Here's how the part is built. I have some questions about the finished solid (model axes, mm). A direction names the side the tool comes from. Give positions to 0.01 mm unless a question says otherwise; leave off trailing zeros. Write each loop counter-clockwise with the first axis right and the second up, starting at its lowest first coordinate (ties: lowest second). Pieces come first, ordered by that corner, then holes. Notation, with made-up numbers: M 54.25,57 L 109.25,57 A25 ccw 109.25,84 Z; hole C 87,-17 d9. An arc over 180 degrees is marked long. Use one line per item in the form item = value. Start each with the question number.
from build123d import *

# Parameters (mm, degrees)
CROQUIS1_R              = 5
CROQUIS1_R_2            = 2.2
SALIENTE_EXTRUIR1_DEPTH = 8
CORTAR_EXTRUIR1_DEPTH   = 26
CROQUIS1_3_R            = 5
CROQUIS1_3_R_2          = 2.65
SALIENTE_EXTRUIR2_DEPTH = 13


with BuildPart() as part:
    # Croquis1 → Saliente-Extruir1 (new body)
    with BuildSketch(Plane(origin=(0, 0, 0), x_dir=(1, 0, 0), z_dir=(0, 1, 0))):
        with BuildLine():
            ThreePointArc((-25, 7), (-24.121320344, 9.121320344), (-22, 10))
            Line((-22, 10), (22, 10))
            ThreePointArc((22, 10), (24.121320344, 9.121320344), (25, 7))
            Line((25, 7), (25, -7))
            ThreePointArc((25, -7), (24.121320344, -9.121320344), (22, -10))
            Line((22, -10), (-22, -10))
            ThreePointArc((-22, -10), (-24.121320344, -9.121320344), (-25, -7))
            Line((-25, -7), (-25, 7))
        make_face()
        with Locations((14.5, 0)):
            Circle(CROQUIS1_R, mode=Mode.SUBTRACT)
        with Locations((-7.5, 0)):
            Circle(CROQUIS1_R_2, mode=Mode.SUBTRACT)
        with Locations((-17.5, 0)):
            Circle(CROQUIS1_R_2, mode=Mode.SUBTRACT)
    extrude(amount=SALIENTE_EXTRUIR1_DEPTH)

    # Croquis2 → Cortar-Extruir1 (cut)
    with BuildSketch(Plane.XY.offset(10)):
        Polygon((4, 8), (5.004091629, 6.995908371), (27.295002856, 6.995908371), (27.295002856, 8), align=None)
    extrude(amount=-CORTAR_EXTRUIR1_DEPTH, mode=Mode.SUBTRACT)

    # Croquis1_3 → Saliente-Extruir2 (add)
    with BuildSketch(Plane(origin=(0, 0, 0), x_dir=(1, 0, 0), z_dir=(0, 1, 0))):
        with Locations((14.5, 0)):
            Circle(CROQUIS1_3_R)
        with Locations((14.5, 0)):
            Circle(CROQUIS1_3_R_2, mode=Mode.SUBTRACT)
    extrude(amount=SALIENTE_EXTRUIR2_DEPTH)


solid = part.part
1) On a 3-axis mill with a long thin cutter (end or side, diameter ignored), from which of +Z, -Z, +X, -X, +Y, -Y can I reach the whole of each face in a straight line? I mean faces 1 (the face through (-10, 8, 0)), 2 (the face through (4.5, 7.5, 0.1)), 3 (the face through (19.27, 9.96, -1.5)). Say none if no direction works.
2) Suppose I cut it at B-B, the plane y = 2.5. List the corners of the cut face in (x, z) for me.
3) Suppose I cut it at D-D, the plane x = 14.5. List the corners of the cut face in (y, z) for me, and give its area (3 significant figures).
4) Suppose I cut it at C-C, the plane z = 0.75. List the corners of the cut face in (x, y) for me.
5) Please list where these lines run through material, in increasing order: line 1 (X direction, y = 3.5, z = 0); line 2 (Z direction, x = -17.5, y = 2.5); line 3 (X direction, y = 5, z = -0.75).
6) Will these pins go through, and if not, where does the flat tip stop? P1, Ø7, axis at x = -7.5, z = 0, coming from the +Y side; P2, Ø2, axis at x = 8, z = 0, coming from the +Y side; P3, Ø2, axis at y = 11.5, z = -2, coming from the -X side.
7) Suppose I cut it at A-A, the plane x = -7.5. List the corners of the cut face in (y, z) for me, and give its area (3 significant figures).
Checks:
q1.face_1 = +Z, -Z, -X, +Y
q1.face_2 = +Z, -Z, +Y
q1.face_3 = +Y
q2.outline = M -25,-7 A3 ccw -22,-10 L 22,-10 A3 ccw 25,-7 L 25,7 A3 ccw 22,10 L -22,10 A3 ccw -25,7 Z; hole C -17.5,0 d4.4; hole C -7.5,0 d4.4; hole C 14.5,0 d5.3
q3.outline = M 0,-10 L 7,-10 L 7,-5 L 13,-5 L 13,-2.65 L 0,-2.65 Z; M 0,2.65 L 13,2.65 L 13,5 L 7,5 L 7,10 L 0,10 Z
q3.area = 131 mm^2
q4.outline = M -25,0 L -19.57,0 L -19.57,8 L -25,8 Z; M -15.43,0 L -9.57,0 L -9.57,8 L -15.43,8 Z; M -5.43,0 L 11.96,0 L 11.96,13 L 9.56,13 L 9.56,7 L 5,7 L 4,8 L -5.43,8 Z; M 17.04,0 L 25,0 L 25,7 L 19.44,7 L 19.44,13 L 17.04,13 Z
q5.line_1 = -25 to -19.7, -15.3 to -9.7, -5.3 to 11.85, 17.15 to 25
q5.line_2 = -10 to -2.2, 2.2 to 10
q5.line_3 = -25 to -19.57, -15.43 to -9.57, -5.43 to 11.96, 17.04 to 25
q6.P1 = 8
q6.P2 = 7
q6.P3 = 9.6
q7.outline = M 0,-10 L 8,-10 L 8,-2.2 L 0,-2.2 Z; M 0,2.2 L 8,2.2 L 8,10 L 0,10 Z
q7.area = 125 mm^2
